Verification items for the finished model (mm, model axes). A direction names the side the tool comes from. Coordinates: 2 decimals unless noted, no trailing zeros. Order: outer loops, then holes, each group sorted by start corner. A loop starts at its lowest first (then second) coordinate and runs counter-clockwise, first axis right, second up. Notation, with made-up numbers: (5.5, -18) -> (31.5, -18) arc R14 ccw to (31.5, -4) -> close; hole circle Ø8 at (-30, -15). An arc over 180 degrees is marked (long way). Write item = value, one per line. Start each with the question number.
from build123d import *

# Parameters (mm, degrees)
F0_W     = 99.06
F0_H     = 99.06
F1_DEPTH = 7.62
F0_W_2   = 114.3
F0_H_2   = 114.3
F2_DEPTH = 88.9
F3_R     = 12.7
F4_DEPTH = 19.127706


with BuildPart() as f1:
    # F0 (on Top) → F1 (new body)
    with BuildSketch(Plane.XY):
        Rectangle(F0_W, F0_H)
    extrude(amount=F1_DEPTH)

    # F0 (on Top) → F2 (join)
    with BuildSketch(Plane.XY):
        Rectangle(F0_W_2, F0_H_2)
        Rectangle(F0_W, F0_H, mode=Mode.SUBTRACT)
    extrude(amount=F2_DEPTH)

    # F3 (on face) → F4 (cut)
    with BuildSketch(Plane.XZ.offset(57.15)):
        with Locations((0, 61.1534)):
            Circle(F3_R)
    extrude(amount=-F4_DEPTH, mode=Mode.SUBTRACT)


solid = f1.part
Item 1: Section check C-C (y = -18.5). Record the boundary of the cut face in (x, z).
Item 2: Tool access check on faces 1 (the flat face through (-1, -57.15, 44)), 2 (the flat face through (49.53, -1, 48)), 3 (the cylindrical face through (-2.753, -53.393, 48.755)). Record the directions out of +Z, -Z, +X, -X, +Y, -Y that give a thin tool (end or side, any length) a straight path to the whole face; none if there is none.
Item 3: Section check A-A (x = 0). Record the boundary of the cut face in (y, z).
Item 4: Gauge pin test, flat ends, axial feed: P1, Ø1, axis at x = 40.5, y = -19.5, coming from the +Z side; P2, Ø12, axis at x = -24, y = -1, coming from the -Z side. Record the tip position at first contact, or that the pin passes through.
Item 5: Thickness scan on line 1 (X direction, y = -8.5, z = 80); line 2 (Z direction, x = 0, y = -53). Record the ranges inside material, lowest first.
Item 6: Section check B-B (z = 14). Record the boundary of the cut face in (x, y).
Item 7: Mould release check, pull along X, two halves, no side actions. Record for faces 4 (the flat face through (-52, 1, 88.9)), 5 (the flat face through (-1, 1, 7.62)), 6 (the flat face through (-57.15, -1, 44)): pulls with the +X half, pulls with the -X half, needs draft (parallel to the pull), parting line crosses it, or undercut.
Filled sheet:
q1.outline = (-57.15, 0) -> (57.15, 0) -> (57.15, 88.9) -> (49.53, 88.9) -> (49.53, 7.62) -> (-49.53, 7.62) -> (-49.53, 88.9) -> (-57.15, 88.9) -> close
q2.face_1 = +Z, -Z, +X, -X, -Y
q2.face_2 = +Z
q2.face_3 = -Y
q3.outline = (-57.15, 0) -> (57.15, 0) -> (57.15, 88.9) -> (49.53, 88.9) -> (49.53, 7.62) -> (-49.53, 7.62) -> (-49.53, 48.45) -> (-57.15, 48.45) -> close; (-57.15, 73.85) -> (-49.53, 73.85) -> (-49.53, 88.9) -> (-57.15, 88.9) -> close
q4.P1 = 7.62
q4.P2 = 0
q5.line_1 = -57.15 to -49.53, 49.53 to 57.15
q5.line_2 = 0 to 48.45, 73.85 to 88.9
q6.outline = (-57.15, -57.15) -> (57.15, -57.15) -> (57.15, 57.15) -> (-57.15, 57.15) -> close; hole (-49.53, -49.53) -> (49.53, -49.53) -> (49.53, 49.53) -> (-49.53, 49.53) -> close
q7.face_4 = needs draft
q7.face_5 = undercut
q7.face_6 = pulls with the -X half
